Geometry: final body of the model. Coordinates: model frame, mm. Face numbers are marked on the shaded views. A direction names the side the tool comes from. Give positions to 0.01 mm unless a question says otherwise; leave off trailing zeros. Loops run counter-clockwise (first coordinate to the right, second up) from the corner with the lowest first, then second, coordinate; pieces in that order, holes last. Notation, with made-up numbers: (74, -11.75) -> (116, -11.75) arc R17 cw to (116, 20.25) -> close; hole circle Ø11 at (-13, -26). An arc over 180 degrees is marked (long way). Answer in a Markdown table with one row per item. Add a question column.
from build123d import *

# Parameters (mm, degrees)
F1_DEPTH = 9
F3_DEPTH = 21
F4_R     = 7.5
F5_DEPTH = 30
F6_W     = 51
F6_H     = 7
F7_DEPTH = 21
F9_DEPTH = 25


with BuildPart() as f1:
    # F0 (on Top) → F1 (new body)
    with BuildSketch(Plane.XY):
        with BuildLine():
            Line((60, 0), (0, 0))
            ThreePointArc((0, 0), (-15, -15), (0, -30))
            Line((0, -30), (60, -30))
            Line((60, -30), (69, -21))
            Line((69, -21), (69, -9))
            Line((69, -9), (60, 0))
        make_face()
    extrude(amount=F1_DEPTH)

    # F2 (on face) → F3 (join)
    with BuildSketch(Plane.XY.offset(9)):
        with BuildLine():
            Line((18, -30), (18, 0))
            Line((18, 0), (0, 0))
            ThreePointArc((0, 0), (-15, -15), (0, -30))
            Line((0, -30), (18, -30))
        make_face()
    extrude(amount=F3_DEPTH)

    # F4 (on face) → F5 (cut)
    with BuildSketch(Plane.XY.offset(30)):
        with Locations((0, -15)):
            Circle(F4_R)
    extrude(amount=-F5_DEPTH, mode=Mode.SUBTRACT)

    # F6 (on face) → F7 (join)
    with BuildSketch(Plane.XY.offset(9)):
        with Locations((43.5, -15)):
            Rectangle(F6_W, F6_H)
    extrude(amount=F7_DEPTH)

    # F8 (on face) → F9 (cut)
    with BuildSketch(Plane.XZ.offset(18.5)):
        Polygon((69, 30), (18, 30), (69, 9), align=None)
    extrude(amount=-F9_DEPTH, mode=Mode.SUBTRACT)


solid = f1.part
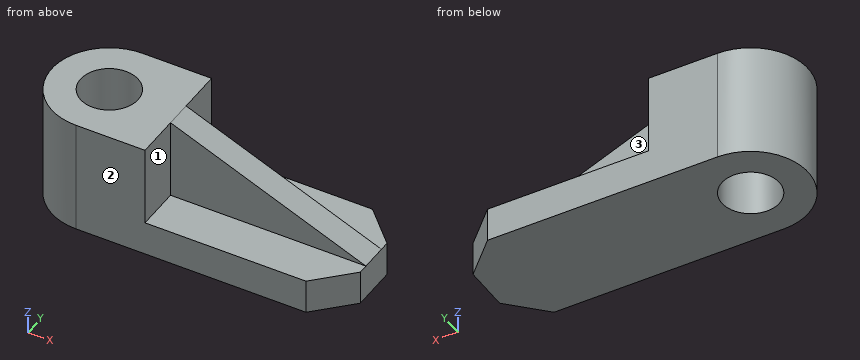
(1) Cut plane C-C on x = -6.5. Return the cut outline in (y, z), then the cut area to 3 significant figures.
(2) Cut plane B-B on z = 16. Return the cut outline in (x, y).
(3) Cut plane D-D on x = 35.5. Return the cut outline in (y, z), then the cut area to 3 significant figures.
(4) Reachability of the marked faces 1, 2 and 3 from +Z, -Z, +X, -X, +Y, -Y: full face, straight path, thin tool, end or side. Return the list, or none.
(5) Material intervals for line 1 along Y through (x, z) = (0, 15.75); line 2 along Z through (x, y) = (40, -27); line 3 along Y through (x, z) = (4.5, 28), sorted ascending. Write a range as from..to.
(6) Pin query (flat end, axial travel): pin 1 Ø1.5 at (x, z) = (18, 4.5) entering from +Y; pin 2 Ø12.5 at (y, z) = (-4, 21) entering from +X; pin 3 Ø2 at (x, z) = (51.5, 16) entering from +Y; pin 4 Ø12 at (x, y) = (28, -18) entering from +Z. Return the tip coordinate at first contact, or that it passes through.
(7) Cut plane A-A on y = -15. Return the cut outline in (x, z), then the cut area to 3 significant figures.
Answer list:
| question | item | result |
|---|---|---|
| 1 | outline | (-28.52, 0) -> (-18.74, 0) -> (-18.74, 30) -> (-28.52, 30) -> close; (-11.26, 0) -> (-1.48, 0) -> (-1.48, 30) -> (-11.26, 30) -> close |
| 1 | area | 587 mm² |
| 2 | outline | (0, -30) -> (18, -30) -> (18, -18.5) -> (52, -18.5) -> (52, -11.5) -> (18, -11.5) -> (18, 0) -> (0, 0) arc R15 ccw to start; hole circle Ø15 at (0, -15) |
| 3 | outline | (-30, 0) -> (0, 0) -> (0, 9) -> (-11.5, 9) -> (-11.5, 22.79) -> (-18.5, 22.79) -> (-18.5, 9) -> (-30, 9) -> close |
| 3 | area | 367 mm² |
| 4 | face 1 | +Z, +X, -Y |
| 4 | face 2 | +Z, -Z, +X, -X, -Y |
| 4 | face 3 | +Z, +X, +Y |
| 5 | line 1 | y = -30..-22.5, -7.5..0 |
| 5 | line 2 | z = 0..9 |
| 5 | line 3 | y = -30..-21, -9..0 |
| 6 | pin 1 | stops at y = 0 |
| 6 | pin 2 | stops at x = 18 |
| 6 | pin 3 | stops at y = -11.5 |
| 6 | pin 4 | stops at z = 28.35 |
| 7 | outline | (-15, 0) -> (-7.5, 0) -> (-7.5, 30) -> (-15, 30) -> close; (7.5, 0) -> (69, 0) -> (69, 9) -> (18, 30) -> (7.5, 30) -> close |
| 7 | area | 1,530 mm² |
